Model file for the job. Use its own axes, mm. Face numbers are marked on the shaded views. A direction names the side the tool comes from. Round coordinates to 2 decimals unless told otherwise and drop trailing zeros. Loops run counter-clockwise (first coordinate to the right, second up) from the corner with the lowest first, then second, coordinate; pieces in that order, holes last. Notation, with made-up numbers: (-30.75, -9) -> (17.25, -9) arc R8 ccw to (17.25, 3) -> close; hole circle Ø8 at (-5.75, 53). An arc over 180 degrees is marked (long way). Use a Markdown table: item, result. Add a question column.
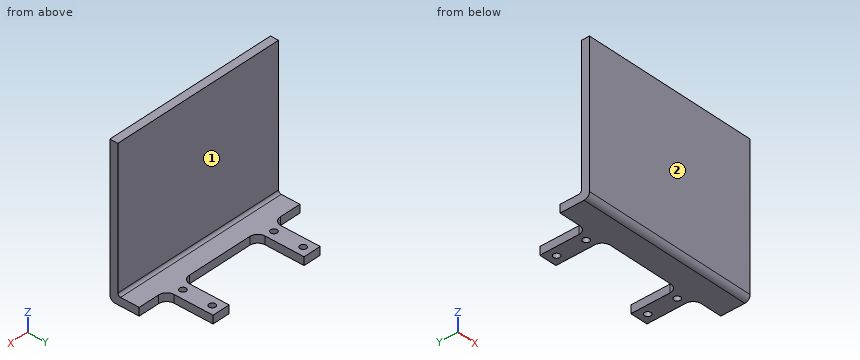
Autodesk Inventor part; units mm, degrees
ref_plane "YZ Plane" through (0, 0, 0) normal (1, 0, 0) x (0, 1, 0)
ref_plane "XZ Plane" through (0, 0, 0) normal (0, 1, 0) x (-1, 0, 0)
ref_plane "XY Plane" through (0, 0, 0) normal (0, 0, 1) x (1, 0, 0)
sketch "草圖1" plane through (0, 0, 0) normal (0, 0, 1) x (1, 0, 0)
  line L0 (0, 0) -> (0, 117.5667) construction
  line L1 (-139.2449, 0) -> (139.2449, 0) construction
  line L2 (-110, 88) -> (-77, 88)
  line L3 (-77, 88) -> (-77, 0)
  line L4 (-77, 0) -> (-110, 0)
  line L5 (-110, 0) -> (-110, 88)
  line L6 (77, 88) -> (110, 88)
  line L7 (110, 88) -> (110, 0)
  line L8 (110, 0) -> (77, 0)
  line L9 (77, 0) -> (77, 88)
  line L10 (-110, 0) -> (-77, 0)
  line L11 (-77, 0) -> (-77, -55)
  line L12 (-77, -55) -> (-110, -55)
  line L13 (-110, -55) -> (-110, 0)
  line L14 (77, 0) -> (110, 0)
  line L15 (110, 0) -> (110, -55)
  line L16 (110, -55) -> (77, -55)
  line L17 (77, -55) -> (77, 0)
  dimension "d0" = 33
  dimension "d1" = 33
  dimension "d2" = 220
  dimension "d3" = 110
  dimension "d4" = 88
  dimension "d5" = 88
  dimension "d6" = 55
  dimension "d7" = 55
extrude "擠出1" add sketch "草圖1" along normal blind 15
sketch "草圖2" plane through (0, 0, 15) normal (0, 0, 1) x (1, 0, 0)
  line L0 (-77, -55) -> (-110, -55) construction
  line L1 (-110, -55) -> (-110, 88) construction
  line L2 (-110, 88) -> (-77, 88) construction
  line L3 (-77, 88) -> (-77, -55) construction
  line L4 (77, 88) -> (110, 88) construction
  line L5 (110, 88) -> (110, -55) construction
  line L6 (110, -55) -> (77, -55) construction
  line L7 (77, -55) -> (77, 88) construction
  line L8 (-110, -55) -> (110, -55)
  line L9 (110, -55) -> (110, -40)
  line L10 (110, -40) -> (-110, -40)
  line L11 (-110, -40) -> (-110, -55)
  point P0 (0, 0)
  dimension "d10" = 15
extrude "擠出2" add sketch "草圖2" along normal blind 260
sketch "草圖3" plane through (0, 0, 15) normal (0, 0, 1) x (1, 0, 0)
  circle A0 centre (-93.5, 71.5) radius 6
  circle A1 centre (-93.5, 16.5) radius 6
  circle A2 centre (93.5, 71.5) radius 6
  circle A3 centre (93.5, 16.5) radius 6
  line L0 (110, 88) -> (77, 88) construction
  line L1 (-77, 88) -> (-110, 88) construction
  line L2 (-93.5, 88) -> (-93.5, -40) construction
  line L3 (-110, -40) -> (-77, -40) construction
  line L4 (93.5, 88) -> (93.5, -40) construction
  line L5 (110, -40) -> (-110, -40) construction
  point P0 (0, 0)
  dimension "d13" = 55
  dimension "d14" = 12
  dimension "d15" = 12
  dimension "d16" = 12
  dimension "d17" = 12
  dimension "d18" = 55
  dimension "d19" = 16.5
  dimension "d20" = 16.5
extrude "擠出3" cut sketch "草圖3" against normal blind 200
sketch "草圖4" plane through (-110, -55, 0) normal (0, -1, 0) x (1, 0, 0)
  line L0 (187, 15) -> (33, 15) construction
  line L1 (33, 15) -> (33, 0) construction
  line L2 (33, 0) -> (0, 0) construction
  line L3 (0, 0) -> (0, 275) construction
  line L4 (0, 275) -> (220, 275) construction
  line L5 (220, 275) -> (220, 0) construction
  line L6 (220, 0) -> (187, 0) construction
  line L7 (187, 0) -> (187, 15) construction
  line L8 (-55, 275) -> (275, 275)
  line L9 (275, 275) -> (275, 15)
  line L10 (275, 15) -> (-55, 15)
  line L11 (-55, 15) -> (-55, 275)
  point P0 (110, 0)
  point P1 (110, 275)
  point P2 (110, 15)
  dimension "d23" = 55
extrude "擠出4" add sketch "草圖4" against normal blind 15
sketch "草圖5" plane through (0, 0, 15) normal (0, 0, -1) x (-1, 0, 0)
  circle A0 centre (-93.5, 71.5) radius 6 construction
  circle A1 centre (93.5, 71.5) radius 6 construction
  circle A2 centre (-93.5, 16.5) radius 6 construction
  circle A3 centre (93.5, 16.5) radius 6 construction
  line L0 (-110, 88) -> (-77, 88) construction
  line L1 (-77, 88) -> (-77, -40) construction
  line L2 (-77, -40) -> (77, -40) construction
  line L3 (77, -55) -> (77, -40) construction
  line L4 (77, -55) -> (-77, -55) construction
  line L5 (-77, -55) -> (-110, -55) construction
  line L6 (-110, -55) -> (-110, -40) construction
  line L7 (-110, -40) -> (-77, -40) construction
  line L8 (-110, -40) -> (-110, 88) construction
  line L9 (-165, -40) -> (-110, -40) construction
  line L10 (-165, -55) -> (-165, -40) construction
  line L11 (-110, -55) -> (-165, -55) construction
  line L12 (-77, -40) -> (-77, -55) construction
  line L13 (77, -40) -> (110, -40) construction
  line L14 (110, -40) -> (110, -55) construction
  line L15 (165, -55) -> (110, -55) construction
  line L16 (165, -40) -> (165, -55) construction
  line L17 (110, -40) -> (165, -40) construction
  line L18 (110, 88) -> (110, -40) construction
  line L19 (77, 88) -> (110, 88) construction
  line L20 (77, -40) -> (77, 88) construction
  line L21 (110, -55) -> (77, -55) construction
  line L22 (-165, -55) -> (165, -55)
  line L23 (165, -55) -> (165, 0)
  line L24 (165, 0) -> (-165, 0)
  line L25 (-165, 0) -> (-165, -55)
  line L26 (165, -55) -> (165, -40)
  point P0 (0, 0)
  dimension "d26" = 40
extrude "擠出5" add sketch "草圖5" along normal blind 15
fillet "圓角1" radius 10 1 edges at (0, -55, 0)
fillet "圓角2" radius 5 1 edges at (0, -40, 15)
fillet "圓角3" radius 15 4 edges at (-77, 0, 7.5) (-110, 0, 7.5) (77, 0, 7.5) (110, 0, 7.5)
equation "\"d3\" = 0.5 * d2"
equation "\"d15\" = d14"
equation "\"d16\" = d14"
equation "\"d17\" = d14"
equation "\"d18\" = d13"
equation "\"d20\" = d19"
1) Tool access for the marked faces 1 and 2: list every direction of +Z, -Z, +X, -X, +Y, -Y with a clear straight run to the whole face (end or side of a thin tool).
2) Pin check, flat tips, straight feed: pin 1 Ø8 at (x, z) = (32.5, 241.5) entering from +Y; pin 2 Ø16.5 at (x, z) = (-12.5, 10) entering from +Y; pin 3 Ø19 at (x, y) = (-93.5, 16.5) entering from +Z. Stop position of each tip, or through.
3) Cut at A-A on x = -93.5. Write the cut outline in (y, z), and give its area (3 significant figures).
4) Wall check: probe 1 along X at (y, z) = (16, 10); probe 2 along Y at (x, z) = (-93.5, 10); probe 3 along Y at (x, z) = (93.5, 4.5). Give the ranges that are in metal, low to high. Write a range as from..to.
5) Cut at B-B on y = 71.5. Write the cut outline in (x, z).
6) Cut at D-D on x = -22.5. Write the cut outline in (y, z), and give its area (3 significant figures).
7) Cut at C-C on y = 5. Write the cut outline in (x, z).
Established:
| question | item | result |
|---|---|---|
| 1 | face 1 | +Z, +X, -X, +Y |
| 1 | face 2 | +Z, -Z, +X, -X, -Y |
| 2 | pin 1 | stops at y = -40 |
| 2 | pin 2 | stops at y = 0 |
| 2 | pin 3 | stops at z = 15 |
| 3 | outline | (-55, 10) arc R10 ccw to (-45, 0) -> (10.5, 0) -> (10.5, 15) -> (-35, 15) arc R5 cw to (-40, 20) -> (-40, 275) -> (-55, 275) -> close; (22.5, 0) -> (65.5, 0) -> (65.5, 15) -> (22.5, 15) -> close; (77.5, 0) -> (88, 0) -> (88, 15) -> (77.5, 15) -> close |
| 3 | area | 5,670 mm^2 |
| 4 | probe 1 | x = -110..-99.48, -87.52..-77, 77..87.52, 99.48..110 |
| 4 | probe 2 | y = -55..10.5, 22.5..65.5, 77.5..88 |
| 4 | probe 3 | y = -53.35..10.5, 22.5..65.5, 77.5..88 |
| 5 | outline | (-110, 0) -> (-99.5, 0) -> (-99.5, 15) -> (-110, 15) -> close; (-87.5, 0) -> (-77, 0) -> (-77, 15) -> (-87.5, 15) -> close; (77, 0) -> (87.5, 0) -> (87.5, 15) -> (77, 15) -> close; (99.5, 0) -> (110, 0) -> (110, 15) -> (99.5, 15) -> close |
| 6 | outline | (-55, 10) arc R10 ccw to (-45, 0) -> (0, 0) -> (0, 15) -> (-35, 15) arc R5 cw to (-40, 20) -> (-40, 275) -> (-55, 275) -> close |
| 6 | area | 4,710 mm^2 |
| 7 | outline | (-113.82, 0) -> (-73.18, 0) -> (-73.18, 15) -> (-113.82, 15) -> close; (73.18, 0) -> (113.82, 0) -> (113.82, 15) -> (73.18, 15) -> close |
